from build123d import *

# Parameters (mm, degrees)
F1_DEPTH = 19.05
F3_R     = 2.29653
F4_DEPTH = 5.588
F2_R     = 2.052631
F5_DEPTH = 5.842


with BuildPart() as f1:
    # F0 (on Front) → F1 (new body)
    with BuildSketch(Plane.XZ):
        with BuildLine():
            Line((60.027805, 1.9), (11.752726, 1.9))
            Line((11.752726, 1.9), (29.430396, 19.57767))
            Line((29.430396, 19.57767), (28.086893, 20.921172))
            Line((28.086893, 20.921172), (10.409223, 3.243503))
            ThreePointArc((10.409223, 3.243503), (9.906439, 1.65845), (10.027805, 0))
            Line((10.027805, 0), (60.027805, 0))
            Line((60.027805, 0), (60.027805, 1.9))
        make_face()
    extrude(amount=F1_DEPTH)

    # F3 (on face) → F4 (cut)
    with BuildSketch(Plane(origin=(3.58286, 0, -3.58286), x_dir=(0, -1, 0), z_dir=(-0.707107, 0, 0.707107))):
        with Locations((14.55, 27.153935)):
            Circle(F3_R)
        with Locations((5.83333, 27.153935)):
            Circle(F3_R)
    extrude(amount=-F4_DEPTH, mode=Mode.SUBTRACT)

    # F2 (on Top) → F5 (cut)
    with BuildSketch(Plane.XY):
        with Locations((28.080662, -10.191665)):
            Circle(F2_R)
    extrude(amount=F5_DEPTH, mode=Mode.SUBTRACT)


solid = f1.part
Input: part model. Units: mm. Frame: model coordinates. A direction names the side the tool comes from. Give positions to 0.01 mm unless a question says otherwise; leave off trailing zeros. Order: outer loops, then holes, each group sorted by start corner. A loop starts at its lowest first (then second) coordinate and runs counter-clockwise, first axis right, second up. Notation, with made-up numbers: (-34.75, -1) - (-21.75, -1) arc R23 ccw to (-21.75, 36) - close; hole circle Ø3 at (40, 27.25). An arc over 180 degrees is marked (long way). Answer as a JSON object with one key per item and string values. Group by question number.
Q1. Cut plane C-C, the plane x = 32. Output: boundary loops of the cut face in (y, z).
Q2. Cut plane B-B, the plane x = 19. Output: boundary loops of the cut face in (y, z), then the cut area to 3 significant figures.
Q3. First-contact query: pin 1 Ø1.5 at (x, y) = (37, -13) entering from -Z; pin 2 Ø3.5 at (x, y) = (28.08, -10.19) entering from -Z; pin 3 Ø8 at (x, z) = (45, 9.5) entering from -Y; pin 4 Ø5.5 at (x, y) = (25.5, -9) entering from +Z. Flat tips, straight axial feed; report the tip coordinate or a pass-through.
Q4. Cut plane D-D, the plane y = -7.5. Output: boundary loops of the cut face in (x, z), then the cut area to 3 significant figures.
Q5. Line query: probe 1 along Z at (x, y) = (56, -2); probe 2 along Z at (x, y) = (28, -7); probe 3 along Z at (x, y) = (19, -15). Output: solid intervals per line, ascending.
Q6. Mould query, pull axis Y, two halves, no side actions, for faces 3 (the face through (29, 0, 1)), 4 (the face through (26.57, -8.8, 0.94)), 5 (the face through (21.86, -5.34, 13.37)), 6 (the face through (60.028, -9, 1)). Classes: pulls with the +Y half, pulls with the -Y half, needs draft (parallel to the pull), parting line crosses it, or undercut.
Q7. Set-up query: faces 1 (the face through (9.91, -9.39, 1.68)), 2 (the face through (36, -9, 1.9)). Return all of +Z, -Z, +X, -X, +Y, -Y with unobstructed straight access to the full face (end or side cutting, diameter ignored); none if empty.
Q8. Cut plane A-A, the plane y = -14.25. Output: boundary loops of the cut face in (x, z), then the cut area to 3 significant figures.
Results:
{
 "1": {"outline": "(-19.05, 0) - (0, 0) - (0, 1.9) - (-19.05, 1.9) - close"},
 "2": {"outline": "(-19.05, 0) - (0, 0) - (0, 1.9) - (-19.05, 1.9) - close; (-19.05, 9.15) - (0, 9.15) - (0, 11.83) - (-19.05, 11.83) - close", "area": "87.4 mm^2"},
 "3": {"pin 1": "z = 0", "pin 2": "z = 16.48", "pin 3": "through", "pin 4": "z = 20.92"},
 "4": {"outline": "(10.03, 0) - (60.03, 0) - (60.03, 1.9) - (11.75, 1.9) - (23.01, 13.16) - (21.67, 14.5) - (10.41, 3.24) arc R4.4 ccw to start; (23.9, 16.74) - (25.24, 15.39) - (29.43, 19.58) - (28.09, 20.92) - close", "area": "138 mm^2"},
 "5": {"probe 1": "0 to 1.9", "probe 2": "0 to 1.9, 18.15 to 20.83", "probe 3": "0 to 1.9, 9.15 to 11.83"},
 "6": {"face 3": "pulls with the +Y half", "face 4": "undercut", "face 5": "undercut", "face 6": "needs draft"},
 "7": {"face 1": "-X, +Y, -Y", "face 2": "+X, +Y, -Y"},
 "8": {"outline": "(10.03, 0) - (60.03, 0) - (60.03, 1.9) - (11.75, 1.9) - (22.52, 12.66) - (21.17, 14.01) - (10.41, 3.24) arc R4.4 ccw to start; (24.39, 17.23) - (25.74, 15.88) - (29.43, 19.58) - (28.09, 20.92) - close", "area": "135 mm^2"}
}
